```python
from build123d import *

# Parameters (mm, degrees)
REDONDEO1_R   = 2
REDONDEO2_R   = 1
REDONDEO3_R   = 0.5
CHAFL_N1_SIZE = 0.5


with BuildPart() as part:
    # Croquis2 → Revolución1 (revolve)
    with BuildSketch(Plane.XY):
        Polygon((0, 0), (25, 0), (17, 17), (8, 17), (8, 16), (4, 16), (4, 64), (0, 64), align=None)
    revolve(axis=Axis((0, 64, 0), (0, -1, 0)))

    # Redondeo1
    redondeo1_edges = [part.edges().sort_by_distance(p)[0] for p in [
        (-17, 17, 0),
        (-25, 0, 0),
    ]]
    fillet(redondeo1_edges, radius=REDONDEO1_R)

    # Redondeo2
    redondeo2_edges = [part.edges().sort_by_distance(p)[0] for p in [
        (-4, 16, 0),
    ]]
    fillet(redondeo2_edges, radius=REDONDEO2_R)

    # Redondeo3
    redondeo3_edges = [part.edges().sort_by_distance(p)[0] for p in [
        (-8, 17, 0),
    ]]
    fillet(redondeo3_edges, radius=REDONDEO3_R)

    # Chaflán1
    chafl_n1_edges = [part.edges().sort_by_distance(p)[0] for p in [
        (-4, 64, 0),
    ]]
    chamfer(chafl_n1_edges, length=CHAFL_N1_SIZE)


solid = part.part
```
Model file for the job. Use its own axes, mm. A direction names the side the tool comes from. Round coordinates to 2 decimals unless told otherwise and drop trailing zeros. Write each loop counter-clockwise with the first axis right and the second up, starting at its lowest first coordinate (ties: lowest second). Pieces come first, ordered by that corner, then holes. Notation, with made-up numbers: M 82.5,32 L 117.5,32 A25 cw 117.5,50 Z; hole C -7.75,-20.75 d6. An arc over 180 degrees is marked long. Put each result on its own line as item: value.
Item 1: Tool access for faces 1 (the flat face through (0, 0, 0)), 2 (the flat face through (7, 17, -7)): list every direction of +Z, -Z, +X, -X, +Y, -Y with a clear straight run to the whole face (end or side of a thin tool).
Responses:
face 1: +Z, -Z, +X, -X, -Y
face 2: +Y
Item 2: Cut at B-B (z = 0). List the corners of the cut face in (x, y).
Responses:
outline: M -23.66,2.85 A2 ccw -21.85,0 L 21.85,0 A2 ccw 23.66,2.85 L 17.54,15.85 A2 ccw 15.73,17 L 8.5,17 A0.5 ccw 8,16.5 L 8,16 L 5,16 A1 cw 4,17 L 4,63.5 L 3.5,64 L -3.5,64 L -4,63.5 L -4,17 A1 cw -5,16 L -8,16 L -8,16.5 A0.5 ccw -8.5,17 L -15.73,17 A2 ccw -17.54,15.85 Z
Item 3: Mould opens along X. For faces 3 (the cylindrical face through (-1.73, 16.25, -7.81)), 4 (the flat face through (-0.1, 16, -5.2)), 5 (the flat face through (0, 64, 0)), 6 (the cylindrical face through (-0.867, 40.576, -3.905)) say: +X half, -X half, draft (parallel to the pull), parting line (faces both ways), or undercut.
Responses:
face 3: undercut
face 4: undercut
face 5: draft
face 6: parting line
Item 4: Flat gauge pins, fed straight in: P1, Ø12, axis at y = 28.5, z = 10.5, coming from the -X side; P2, Ø8, axis at x = -0.5, y = 36.5, coming from the +Z side; P3, Ø10, axis at x = -5.5, y = 17, coming from the +Z side; P4, Ø6, axis at x = 18.5, z = -18.5, coming from the +Y side. Where does each tip first touch, or does it go through?
Responses:
P1: through
P2: z = 4
P3: z = 18.84
P4: y = 3.9
Item 5: Probe L1, parallel to Z at x = 0, y = 16.3; L2, parallel to Z at x = 0, y = 16.25; L3, parallel to Y at x = -12.5, z = 7.5. List the from-to ranges inside material, lowest first. Write a range as from..to.
Responses:
L1: -17.25..-8, -4.29..4.29, 8..17.25
L2: -17.29..-8, -4.34..4.34, 8..17.29
L3: 0..17
Item 6: Cut at A-A (x = 0). List the corners of the cut face in (y, z).
Responses:
outline: M 0,-21.85 A2 ccw 2.85,-23.66 L 15.85,-17.54 A2 ccw 17,-15.73 L 17,-8.5 A0.5 ccw 16.5,-8 L 16,-8 L 16,-5 A1 cw 17,-4 L 63.5,-4 L 64,-3.5 L 64,3.5 L 63.5,4 L 17,4 A1 cw 16,5 L 16,8 L 16.5,8 A0.5 ccw 17,8.5 L 17,15.73 A2 ccw 15.85,17.54 L 2.85,23.66 A2 ccw 0,21.85 Z
Item 7: Cut at C-C (y = 22). List the corners of the cut face in (x, z).
Responses:
outline: C 0,0 d8
Item 8: Cut at D-D (y = 10.5). List the corners of the cut face in (x, z).
Responses:
outline: C 0,0 d40.12
